Geometry: final body of the model. Coordinates: model frame, mm. Face numbers are marked on the shaded views. A direction names the side the tool comes from. Give positions to 0.01 mm unless a question says otherwise; leave off trailing zeros. Loops run counter-clockwise (first coordinate to the right, second up) from the corner with the lowest first, then second, coordinate; pieces in that order, holes last. Notation, with made-up numbers: (53.25, -13.5) -> (112.25, -13.5) arc R13 cw to (112.25, 4.5) -> close; hole circle Ø10 at (78, 24.25). An arc over 180 degrees is marked (long way). One line per item, written item: value. Start each with the question number.
from build123d import *

# Parameters (mm, degrees)
CUT_EXTRUDE_1_DEPTH = 6
SKETCH_3_R          = 3.75
EXTRUDE_1_DEPTH     = 3


with BuildPart() as part:
    # 草图1 → 旋转1 (revolve)
    with BuildSketch(Plane.XY, mode=Mode.PRIVATE) as revolve_1_sk:
        with BuildLine():
            Line((-0.856624327, 0), (-2.3, 2.5))
            Line((-2.3, 2.5), (-6, 2.5))
            Line((-6, 2.5), (-6, 4.4))
            ThreePointArc((-6, 4.4), (-5.824264069, 4.824264069), (-5.4, 5))
            Line((-5.4, 5), (0, 5))
            Line((0, 5), (0, 3.4))
            ThreePointArc((0, 3.4), (0.046179295, 3.255234258), (0.167656961, 3.163949955))
            Line((0.167656961, 3.163949955), (0.597656961, 3.013949955))
            ThreePointArc((0.597656961, 3.013949955), (0.638241835, 3.003512159), (0.68, 3))
            Line((0.68, 3), (11.3865, 3))
            Line((11.3865, 3), (12, 2.3865))
            Line((12, 2.3865), (12, 0))
            Line((12, 0), (-0.856624327, 0))
        make_face()
    revolve(revolve_1_sk.sketch.rotate(Axis((12, 0, 0), (-1, 0, 0)), 270), axis=Axis((12, 0, 0), (-1, 0, 0)))

    # 草图2 → 切除-拉伸1 (cut)
    with BuildSketch(Plane(origin=(-2.3, 0, 0), x_dir=(0, 0, -1), z_dir=(1, 0, 0))):
        Polygon((-2.5, 1.443375673), (-2.5, -1.443375673), (0, -2.886751346), (2.5, -1.443375673), (2.5, 1.443375673), (0, 2.886751346), align=None)
    extrude(amount=-CUT_EXTRUDE_1_DEPTH, mode=Mode.SUBTRACT)


with BuildPart() as body_2:
    # 草图3 → 凸台-拉伸1 (new body)
    with BuildSketch(Plane(origin=(0, 0, 0), x_dir=(0, 0, -1), z_dir=(1, 0, 0))):
        Circle(SKETCH_3_R)
    extrude(amount=-EXTRUDE_1_DEPTH)

    # Delete Face 1: 1 face struck out; the rest of the skin is kept as a surface, the solid goes
    delete_face_1_1_drop = [body_2.part.faces().sort_by_distance(Vector(p))[0] for p in ((-3, 0, 0),)]
    delete_face_1_1 = Shell(body_2.part.faces() - delete_face_1_1_drop)


solid = part.part
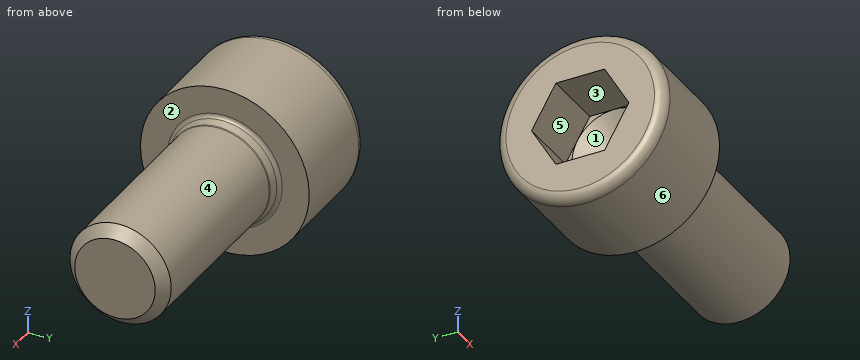
Item 1: Section A-A, the plane x = -2.75. Output: boundary loops of the cut face in (y, z), then the cut area to 3 significant figures.
Item 2: Mould query, pull axis Z, two halves, no side actions, for the marked faces 1, 2, 3 and 4. Classes: pulls with the +Z half, pulls with the -Z half, needs draft (parallel to the pull), parting line crosses it, or undercut.
Item 3: Section B-B, the plane x = 6.5. Output: boundary loops of the cut face in (y, z), then the cut area to 3 significant figures.
Item 4: Pin query (flat end, axial travel): pin 1 (1 mm diameter, centred on x = 9, y = 1.5, fed in from +Z); pin 2 (0.6 mm diameter, centred on y = -2.5, z = 0, fed in from -X); pin 3 (1.5 mm diameter, centred on x = 4.5, y = 0.5, fed in from +Z). Return the tip coordinate at first contact, or that it passes through.
Item 5: Access query for the marked faces 5 and 6. Directions: +Z, -Z, +X, -X, +Y, -Y. A direction counts if a zero-diameter tool reaches every point of the face in a straight line with its end or side. Return the directions, or none.
Item 6: Ray query, line 1 along X through (y, z) = (-4, 1.25); line 2 along Z through (x, y) = (-3.5, 1.25); line 3 along Y through (x, z) = (-4.75, 0.5). Return the intervals inside material, ascending. Write a range as [from, to].
Geometry check:
1. outline: circle Ø10 at (0, 0); hole (-2.89, 0) -> (-1.44, -2.5) -> (1.44, -2.5) -> (2.89, 0) -> (1.44, 2.5) -> (-1.44, 2.5) -> close
1. area: 56.9 mm2
2. face 1: undercut
2. face 2: needs draft
2. face 3: undercut
2. face 4: parting line crosses it
3. outline: circle Ø6 at (0, 0)
3. area: 28.3 mm2
4. pin 1: stops at z = 2.83
4. pin 2: stops at x = -2.3
4. pin 3: stops at z = 3
5. face 5: -X
5. face 6: +X, -X
6. line 1: x = [-6, 0]
6. line 2: z = [-4.84, -2.5], [2.5, 4.84]
6. line 3: y = [-4.97, -2.6], [2.6, 4.97]
